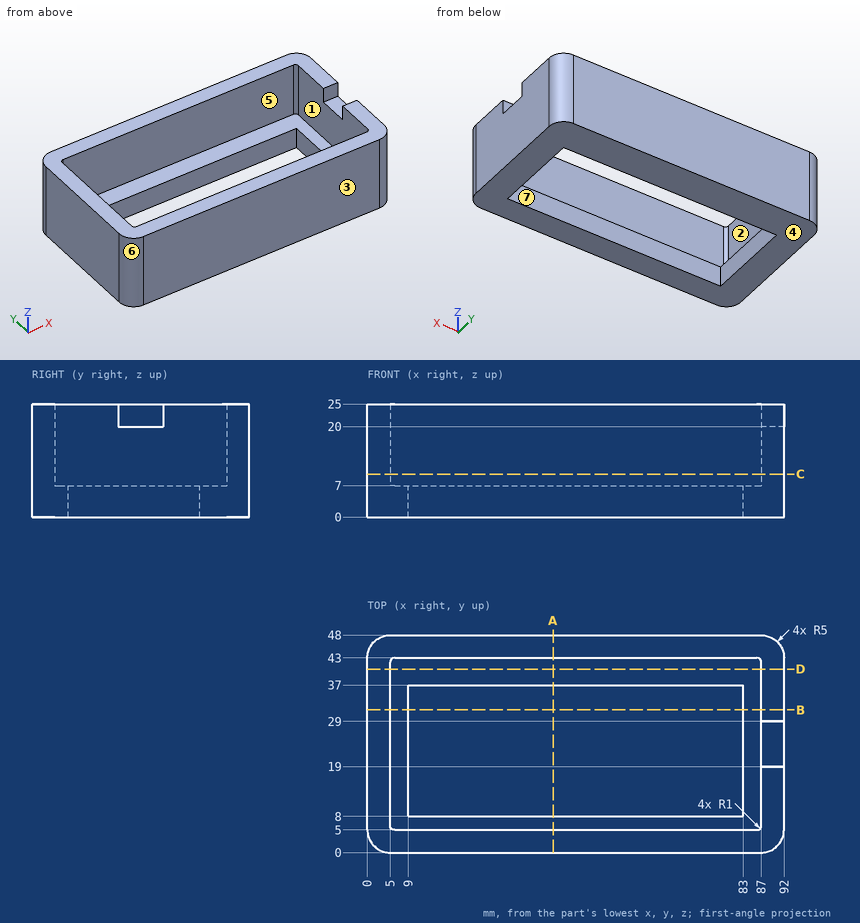
Design review of the part shown in the three views and the two pictorial views. Dimensions are in mm from the part's minimum x, y and z. A direction names the side the tool comes from. Round coordinates to 2 decimals unless told otherwise and drop trailing zeros. Order: outer loops, then holes, each group sorted by start corner. A loop starts at its lowest first (then second) coordinate and runs counter-clockwise, first axis right, second up. Notation, with made-up numbers: (-32, 75) - (27, 75) arc R33 cw to (27, 109) - close; hole circle Ø6 at (73, 27.5). An arc over 180 degrees is marked (long way). One line per question, with ' | ' between items.
Item 1: Take a section at C-C, the plane z = 9.5. Write out the cut boundary in (x, y), then the cut area to 3 significant figures.
Checks:
outline: (0, 5) arc R5 ccw to (5, 0) - (87, 0) arc R5 ccw to (92, 5) - (92, 43) arc R5 ccw to (87, 48) - (5, 48) arc R5 ccw to (0, 43) - close; hole (5, 6) arc R1 ccw to (6, 5) - (86, 5) arc R1 ccw to (87, 6) - (87, 42) arc R1 ccw to (86, 43) - (6, 43) arc R1 ccw to (5, 42) - close | area: 1,280 mm²
Item 2: Take a section at D-D, the plane y = 40.5. Write out the cut boundary in (x, z), then the cut area to 3 significant figures.
Checks:
outline: (0, 0) - (92, 0) - (92, 25) - (87, 25) - (87, 7) - (5, 7) - (5, 25) - (0, 25) - close | area: 824 mm²
Item 3: For P1, Ø4, axis at x = 89, z = 23.5, coming from the -Y side; P2, Ø19, axis at x = 33, y = 15.5, coming from the +Z side; P3, Ø4, axis at x = 90.5, z = 21.5, coming from the +Y side; P4, Ø4, axis at x = 90.5, y = 26, coming from the +Z side, all flat-tipped, find the tip position at first contact; note any pin that passes through.
Checks:
P1: y = 0 | P2: z = 7 | P3: y = 47.77 | P4: z = 20
Item 4: Machinability: for the marked faces 5, 6 and 7, which of the approach directions +Z, -Z, +X, -X, +Y, -Y give a long, thin tool a straight path to every point of the face, cutting with its end or side? Answer none if there is none.
Checks:
face 5: +Z | face 6: +Z, -Z, -X, -Y | face 7: +Z, -Z
Item 5: Take a section at B-B, the plane y = 31.5. Write out the cut boundary in (x, z), then the cut area to 3 significant figures.
Checks:
outline: (0, 0) - (9, 0) - (9, 7) - (5, 7) - (5, 25) - (0, 25) - close; (83, 0) - (92, 0) - (92, 25) - (87, 25) - (87, 7) - (83, 7) - close | area: 306 mm²
Item 6: Wall thickness on line 1 (Y direction, x = 56, z = 19.75); line 2 (X direction, y = 41, z = 12.5); line 3 (X direction, y = 9, z = 6.75): over which ranges is each line inside the solid? List them lowest first. Write a range as [from, to].
Checks:
line 1: [0, 5], [43, 48] | line 2: [0, 5], [87, 92] | line 3: [0, 9], [83, 92]
Item 7: Draft analysis for pull direction Y (two halves, no side actions). For the marked faces 1, 2, 3 and 4, state which applies: +Y half, -Y half, draft (parallel to the pull), parting line (faces both ways), or undercut.
Checks:
face 1: undercut | face 2: undercut | face 3: -Y half | face 4: draft
Item 8: Take a section at A-A, the plane x = 41. Write out the cut boundary in (y, z), then the cut area to 3 significant figures.
Checks:
outline: (0, 0) - (8, 0) - (8, 7) - (5, 7) - (5, 25) - (0, 25) - close; (37, 0) - (48, 0) - (48, 25) - (43, 25) - (43, 7) - (37, 7) - close | area: 313 mm²
